The model under review builds one solid part; all positions refer to its coordinate system, in mm. Coordinates: 2 decimals unless noted, no trailing zeros. Write each loop counter-clockwise with the first axis right and the second up, starting at its lowest first coordinate (ties: lowest second). Pieces come first, ordered by that corner, then holes. Notation, with made-up numbers: (28, -18.75) -> (58, -18.75) arc R17 ccw to (58, 13.25) -> close; hole circle Ø5 at (22, 3). An arc over 180 degrees is marked (long way). Put each result on its own line as item: value. Start each with the question number.
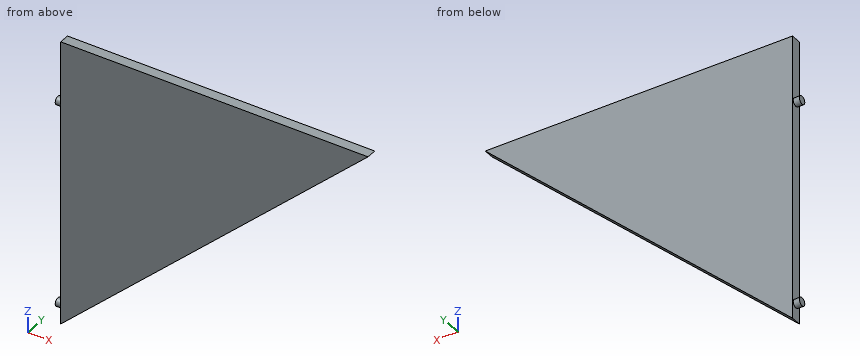
from build123d import *

# Parameters (mm, degrees)
BOSS_EXTRUDE1_DEPTH = 5
SKETCH2_R           = 2
BOSS_EXTRUDE2_DEPTH = 3


with BuildPart() as part:
    # Sketch1 → Boss-Extrude1 (new body)
    with BuildSketch(Plane(origin=(0, 0, 0), x_dir=(1, 0, 0), z_dir=(0, 1, 0))):
        Polygon((-50.263774427, 46.912856132), (99.736225573, -93.087143868), (-50.263774427, -93.087143868), align=None)
    extrude(amount=BOSS_EXTRUDE1_DEPTH)

    # Sketch2 → Boss-Extrude2 (add)
    with BuildSketch(Plane.ZY.offset(50.263774427)):
        with Locations((-38.421386897, 2.5)):
            Circle(SKETCH2_R)
        with Locations((61.578613103, 2.5)):
            Circle(SKETCH2_R)
    extrude(amount=BOSS_EXTRUDE2_DEPTH)


solid = part.part
1. Consider section A-A on y = 2.5. State the section outline as (x, z) points, then the cut area to 3 significant figures.
2. Consider section C-C on x = 59. State the section outline as (y, z) points.
3. Wall thickness on line 1 (Z direction, x = 0, y = 1.5); line 2 (X direction, y = 0.9, z = 59.5); line 3 (Z direction, x = 61.5, y = 2.1): over which ranges is each line inside the solid? List them lowest first. Write a range as from..to.
4. Insertion check: P1, Ø1, axis at y = 3.5, z = 76, coming from the -X side. The pin has a flat end and moves straight along its axis. Give the tip position at first contact, or say it passes through.
5. Consider section B-B on z = 0. State the section outline as (x, y) points, then the cut area to 3 significant figures.
Output values:
1. outline: (-53.26, -40.42) -> (-50.26, -40.42) -> (-50.26, -46.91) -> (99.74, 93.09) -> (-50.26, 93.09) -> (-50.26, 63.58) -> (-53.26, 63.58) -> (-53.26, 59.58) -> (-50.26, 59.58) -> (-50.26, -36.42) -> (-53.26, -36.42) -> close
1. area: 10,500 mm^2
2. outline: (0, 55.07) -> (5, 55.07) -> (5, 93.09) -> (0, 93.09) -> close
3. line 1: z = 0..93.09
3. line 2: x = -50.26..63.75
3. line 3: z = 57.4..93.09
4. P1: stops at x = -50.26
5. outline: (-50.26, 0) -> (0, 0) -> (0, 5) -> (-50.26, 5) -> close
5. area: 251 mm^2
